Check sheet for the drawn part. Datum: minimum x, y, z corner. Units: mm. Coordinates: 2 decimals unless noted, no trailing zeros. Order: outer loops, then holes, each group sorted by start corner. A loop starts at its lowest first (then second) coordinate and runs counter-clockwise, first axis right, second up.
1. Thickness scan on line 1 (Y direction, x = 14.75, z = 90.5); line 2 (X direction, y = 16.5, z = 52); line 3 (X direction, y = 26.5, z = 69). Record the ranges inside material, lowest first.
2. Gauge pin test, flat ends, axial feed: pin 1 Ø12 at (y, z) = (22, 38.5) entering from -X; pin 2 Ø1.5 at (y, z) = (10, 38) entering from +X; pin 3 Ø1.1 at (x, y) = (16, 29.5) entering from -Z. Record the tip position at first contact, or that the pin passes through.
3. Cross-section at A-A (x = 15). Enter the section's corners in (y, z).
4. Cross-section at C-C (z = 34.5). Enter the section's corners in (x, y).
5. Cross-section at B-B (z = 73.5). Enter the section's corners in (x, y).
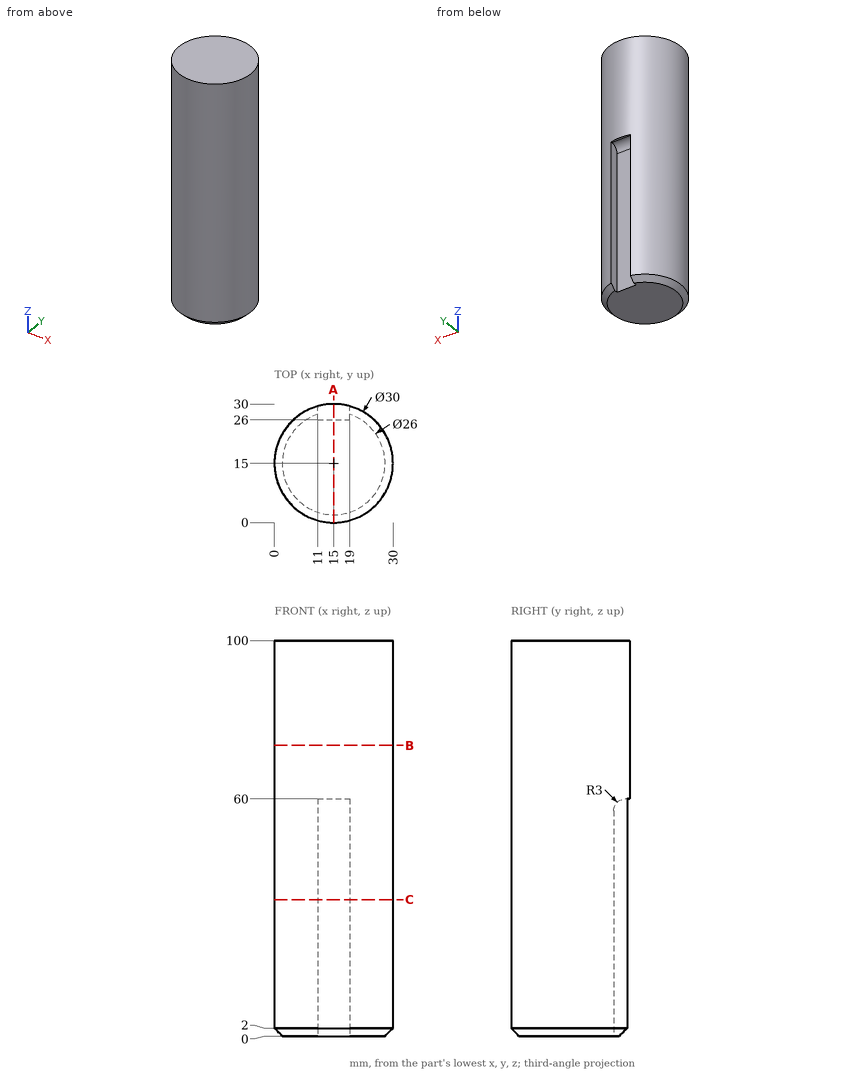
Data:
1. line 1: y = 0 to 30
1. line 2: x = 0.08 to 29.92
1. line 3: x = 5.37 to 24.63
2. pin 1: stops at x = 0.03
2. pin 2: stops at x = 29.39
2. pin 3: stops at z = 60
3. outline: (0, 2) - (2, 0) - (26, 0) - (26, 57) arc R3 cw to (29, 60) - (30, 60) - (30, 100) - (0, 100) - close
4. outline: (11, 26) - (11, 29.46) arc R15 ccw (long way) to (19, 29.46) - (19, 26) - close
5. outline: circle Ø30 at (15, 15)
